Part model, mm, in its own coordinate system. A direction names the side the tool comes from. Round coordinates to 2 decimals unless told otherwise and drop trailing zeros. Order: outer loops, then holes, each group sorted by start corner. A loop starts at its lowest first (then second) coordinate and runs counter-clockwise, first axis right, second up. Notation, with made-up numbers: (-5.75, 22.5) - (6.25, 22.5) arc R17 cw to (6.25, 54.5) - close; hole circle Ø8 at (-26.5, 20). An arc over 180 degrees is marked (long way). Return JSON: item names as keys, results as strings. Group by question number.
Item 1: Saw through at A-A on y = -136.5. List the corners of the cut face in (x, z).
Item 2: Saw through at C-C on z = 10. List the corners of the cut face in (x, y).
Item 3: Probe probe 1 along Y at (x, z) = (23.5, 6); probe 2 along Z at (x, y) = (0, -145); probe 3 along X at (y, z) = (-31.5, 12). List the from-to ranges inside material, lowest first.
Item 4: Drop flat-ended pins along their axis: pin 1 (1 mm diameter, centred on x = 35, y = -136, fed in from +Z); pin 2 (8 mm diameter, centred on x = -7, y = -86, fed in from -Z); pin 3 (8 mm diameter, centred on y = -134, z = 45.5, fed in from -X). Give the stop position or say it passes through.
Item 5: Saw through at B-B on x = 35.5. List the corners of the cut face in (y, z), and give its area (3 significant figures).
Item 6: Two-plate mould, pull along Z, no slides. Class faces 1 (the face through (1, -88, 39.169)), 2 (the face through (3, 0, -2)), 3 (the face through (45, -82, -55.492)): released by +Z, released by -Z, zero draft, split by the parting line, or undercut.
Item 7: Saw through at D-D on x = 2. List the corners of the cut face in (y, z), and give its area (3 significant figures).
Item 8: Tool access for faces 4 (the face through (3, -10.16, -7)), 5 (the face through (3, -116, 8.008)), 6 (the face through (44, -139.7, 38)), 7 (the face through (-6.776, -133, 44)): list every direction of +Z, -Z, +X, -X, +Y, -Y with a clear straight run to the whole face (end or side of a thin tool).
```python
from build123d import *

# Parameters (mm, degrees)
F0_W      = 102.0336635411
F0_H      = 104.8214659095
F1_DEPTH  = 177.8
F2_R      = 15.24
F3_T      = -10.16
F4_W      = 13.97
F4_H      = 21.2457677329
F4_H_2    = 26.0814659095
F6_DEPTH  = 40.64
F5_W      = 13.97
F5_H      = 46.4908947945
F7_DEPTH  = 40.64
F8_R      = 15.24
F10_W     = 63.5
F10_H     = 12.7
F11_DEPTH = 91.186


with BuildPart() as f1:
    # F0 (on Front) → F1 (new body)
    with BuildSketch(Plane.XZ):
        with Locations((3.6009196192, -3.0814781785)):
            Rectangle(F0_W, F0_H)
    extrude(amount=F1_DEPTH)

    # F2
    f2_edges = [f1.edges().sort_by_distance(p)[0] for p in [
        (54.617751, -88.9, 49.329255),
    ]]
    fillet(f2_edges, radius=F2_R)

    # F3
    f3_openings = [f1.faces().sort_by_distance(p)[0] for p in [
        (3.60092, -88.9, -55.492211),
    ]]
    offset(amount=F3_T, openings=f3_openings)

    # F4 (on face) → F6 (cut)
    with BuildSketch(Plane.YZ.offset(54.6177513897)):
        with Locations((-132.715, 44.7121386427)):
            Rectangle(F4_W, F4_H)
        with Locations((-132.715, 21.0485218215)):
            Rectangle(F4_W, F4_H_2)
    extrude(amount=-F6_DEPTH, mode=Mode.SUBTRACT)

    # F5 (on face) → F7 (cut)
    with BuildSketch(Plane(origin=(-47.4159121513, 0, 0), x_dir=(0, -1, 0), z_dir=(-1, 0, 0))):
        with Locations((132.715, 31.253236264)):
            Rectangle(F5_W, F5_H)
    extrude(amount=-F7_DEPTH, mode=Mode.SUBTRACT)

    # F8
    f8_edges = [f1.edges().sort_by_distance(p)[0] for p in [
        (-47.415912, -62.865, 49.329255),
        (-47.415912, -158.75, 49.329255),
    ]]
    fillet(f8_edges, radius=F8_R)

    # F10 (on face) → F11 (join)
    with BuildSketch(Plane.YZ.offset(-37.2559121513)):
        with Locations((-115.8445860147, 1.6577888668)):
            Rectangle(F10_W, F10_H)
    extrude(amount=F11_DEPTH)


solid = f1.part
```
Filled in:
{
 "1": {"outline": "(-47.42, -55.49) - (-37.26, -55.49) - (-37.26, -4.69) - (44.46, -4.69) - (44.46, -55.49) - (54.62, -55.49) - (54.62, 8.01) - (-47.42, 8.01) - close; (-6.78, 39.17) - (13.98, 39.17) - (13.98, 49.33) - (-6.78, 49.33) - close"},
 "2": {"outline": "(-47.42, -177.8) - (54.62, -177.8) - (54.62, -139.7) - (44.46, -139.7) - (44.46, -167.64) - (-37.26, -167.64) - (-37.26, -139.7) - (-47.42, -139.7) - close; (-47.42, -125.73) - (-37.26, -125.73) - (-37.26, -10.16) - (44.46, -10.16) - (44.46, -125.73) - (54.62, -125.73) - (54.62, 0) - (-47.42, 0) - close"},
 "3": {"probe 1": "y = -177.8 to -167.64, -147.59 to -84.09, -10.16 to 0", "probe 2": "z = -4.69 to 8.01, 39.17 to 49.33", "probe 3": "x = -47.42 to -37.26, 44.46 to 54.62"},
 "4": {"pin 1": "stops at z = 8.01", "pin 2": "stops at z = -4.69", "pin 3": "stops at x = -6.78"},
 "5": {"outline": "(-177.8, -55.49) - (-167.64, -55.49) - (-167.64, 39.17) - (-139.7, 39.17) - (-139.7, 49.33) - (-177.8, 49.33) - close; (-147.59, -4.69) - (-84.09, -4.69) - (-84.09, 8.01) - (-147.59, 8.01) - close; (-125.73, 39.17) - (-10.16, 39.17) - (-10.16, -55.49) - (0, -55.49) - (0, 49.33) - (-125.73, 49.33) - close", "area": "4,390 mm^2"},
 "6": {"face 1": "undercut", "face 2": "zero draft", "face 3": "released by -Z"},
 "7": {"outline": "(-177.8, -55.49) - (-167.64, -55.49) - (-167.64, 39.17) - (-10.16, 39.17) - (-10.16, -55.49) - (0, -55.49) - (0, 49.33) - (-177.8, 49.33) - close; (-147.59, -4.69) - (-84.09, -4.69) - (-84.09, 8.01) - (-147.59, 8.01) - close", "area": "4,540 mm^2"},
 "8": {"face 4": "-Z", "face 5": "none", "face 6": "+Z, +X", "face 7": "+Z, -X"}
}
